For this review, use the dimensioned drawing (mm, ordinates from the lowest corner) and the shaded views. Round coordinates to 2 decimals unless told otherwise and drop trailing zeros. Write each loop counter-clockwise with the first axis right and the second up, starting at its lowest first coordinate (ties: lowest second). Pieces come first, ordered by that corner, then holes.
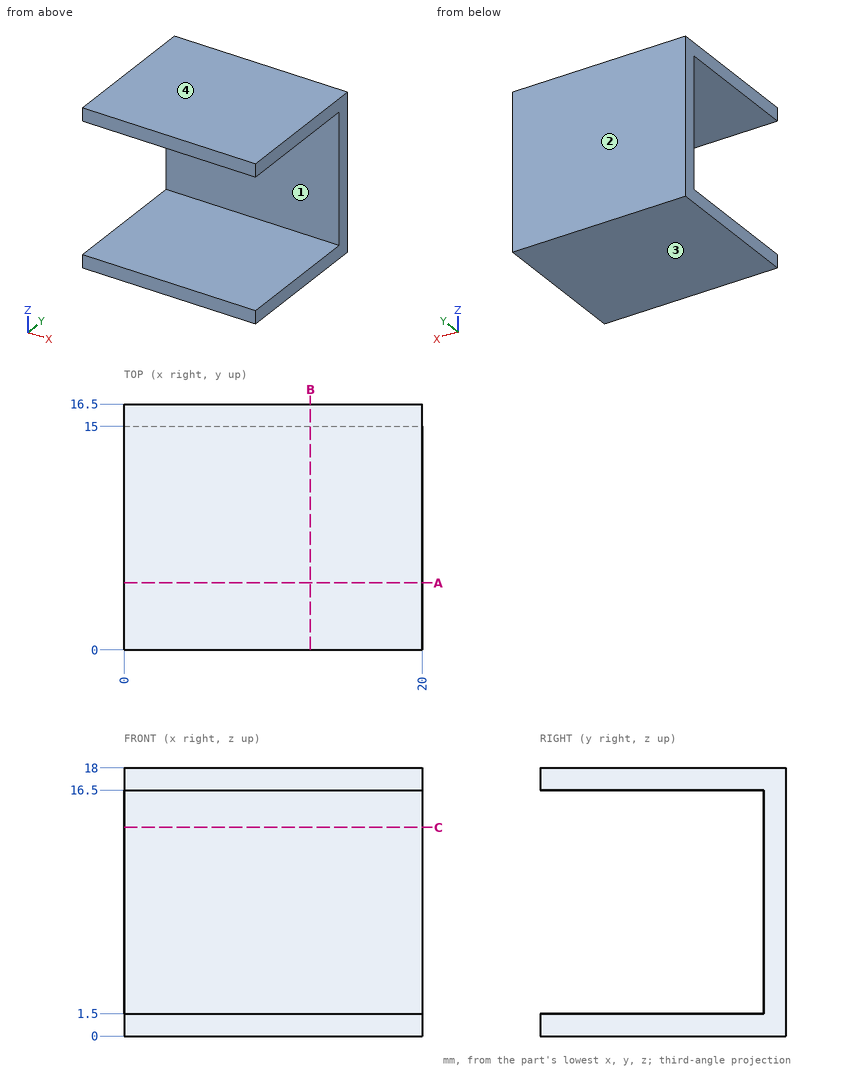
1) Add section C-C on z = 14. State the section outline as (x, y) points, and give its area (3 significant figures).
2) For P1, Ø7.5, axis at x = 7, z = 9.5, coming from the -Y side; P2, Ø3, axis at x = 14.5, y = 2.5, coming from the -Z side, all flat-tipped, find the tip position at first contact; note any pin that passes through.
3) The part is to be moulded in two halves that separate along Z. For the marked faces 1, 2, 3 and 4, say which applies: pulls with the +Z half, pulls with the -Z half, needs draft (parallel to the pull), parting line crosses it, or undercut.
4) Add section B-B on x = 12.5. State the section outline as (y, z) points, and give its area (3 significant figures).
5) Add section A-A on y = 4.5. State the section outline as (x, z) points.
6) For line 1 along Z through (x, y) = (16.25, 3); line 2 along Y through (x, z) = (17.75, 4.75), list the stretches that pass through material, from the lowest coordinate up.
Computed:
1. outline: (0, 15) - (20, 15) - (20, 16.5) - (0, 16.5) - close
1. area: 30.0 mm2
2. P1: stops at y = 15
2. P2: stops at z = 0
3. face 1: undercut
3. face 2: needs draft
3. face 3: pulls with the -Z half
3. face 4: pulls with the +Z half
4. outline: (0, 0) - (16.5, 0) - (16.5, 18) - (0, 18) - (0, 16.5) - (15, 16.5) - (15, 1.5) - (0, 1.5) - close
4. area: 72.0 mm2
5. outline: (0, 0) - (20, 0) - (20, 1.5) - (0, 1.5) - close; (0, 16.5) - (20, 16.5) - (20, 18) - (0, 18) - close
6. line 1: z = 0 to 1.5, 16.5 to 18
6. line 2: y = 15 to 16.5
